Model file for the job. Use its own axes, mm. Face numbers are marked on the shaded views. Coordinates: 2 decimals unless noted, no trailing zeros. Write each loop counter-clockwise with the first axis right and the second up, starting at its lowest first coordinate (ties: lowest second). Pieces come first, ordered by that corner, then holes. Notation, with made-up numbers: (-18, 29) -> (11, 29) arc R15 cw to (11, 45) -> close; hole circle Ø11 at (2, 11). An arc over 180 degrees is marked (long way). Answer as a JSON object with one key per item and string values. Group by question number.
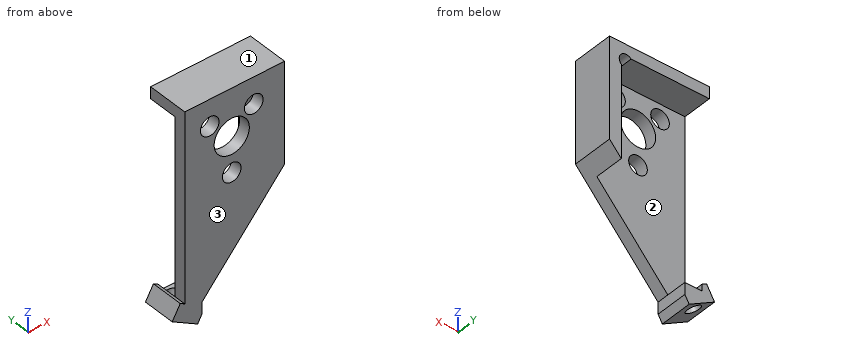
from build123d import *

# Parameters (mm, degrees)
SKETCH1_W                     = 8.5
SKETCH1_H                     = 17.5
BOSS_EXTRUDE1_DEPTH           = 3.5
SKETCH2_W                     = 6.5
SKETCH2_H                     = 15.5
CUT_EXTRUDE1_DEPTH            = 2.5
SKETCH3_R                     = 1.5
GRIN_HOLE_DEPTH               = 2
SKETCH6_R                     = 0.5953125
CORNER_DIVOT_DEPTH            = 2.5
SKETCH7_R                     = 0.79375
MAGNET_HOLES_DEPTH            = 2
BOSS_EXTRUDE2_DEPTH           = 3.5
SKETCH14_W                    = 5.965258944
SKETCH14_H                    = 5.132960456
SET_SCREW_EXTENSION_DEPTH     = 0.75
TAP_DRILL_FOR_0_80_TAP1_D     = 1.19126
TAP_DRILL_FOR_0_80_TAP1_DEPTH = 7.11
TAP_DRILL_FOR_0_80_TAP1_TIP   = 0.357890611
DIAGONAL_CUT_DEPTH            = 5
SKETCH16_W                    = 1
SKETCH16_H                    = 15.5
VERTICAL_CUT_DEPTH            = 3


with BuildPart() as part:
    # Sketch1 → Boss-Extrude1 (new body)
    with BuildSketch(Plane(origin=(0, 0, 0), x_dir=(1, 0, 0), z_dir=(0, 1, 0))):
        Rectangle(SKETCH1_W, SKETCH1_H)
    extrude(amount=BOSS_EXTRUDE1_DEPTH)

    # Sketch2 → Cut-Extrude1 (cut)
    with BuildSketch(Plane(origin=(0, 3.5, 0), x_dir=(1, 0, 0), z_dir=(0, 1, 0))):
        Rectangle(SKETCH2_W, SKETCH2_H)
    extrude(amount=-CUT_EXTRUDE1_DEPTH, mode=Mode.SUBTRACT)

    # Sketch3 → GRIN Hole (cut, through all)
    with BuildSketch(Plane(origin=(0, 1, 0), x_dir=(1, 0, 0), z_dir=(0, 1, 0))):
        with Locations((-0.25, -4.75)):
            Circle(SKETCH3_R)
    extrude(amount=-GRIN_HOLE_DEPTH, mode=Mode.SUBTRACT)

    # Sketch6 → Corner divot (cut)
    with BuildSketch(Plane(origin=(0, 3.5, 0), x_dir=(1, 0, 0), z_dir=(0, 1, 0))):
        with Locations((2.829050494, -7.329050494)):
            Circle(SKETCH6_R)
    extrude(amount=-CORNER_DIVOT_DEPTH, mode=Mode.SUBTRACT)

    # Sketch7 → Magnet Holes (cut, through all)
    with BuildSketch(Plane(origin=(0, 1, 0), x_dir=(1, 0, 0), z_dir=(0, 1, 0))):
        with Locations((-0.25, -1.75)):
            Circle(SKETCH7_R)
        with Locations((-2.125, -6.5)):
            Circle(SKETCH7_R)
        with Locations((1.625, -6.5)):
            Circle(SKETCH7_R)
    extrude(amount=-MAGNET_HOLES_DEPTH, mode=Mode.SUBTRACT)

    # Sketch9 → Boss-Extrude2 (add)
    with BuildSketch(Plane(origin=(0, 3.5, 0), x_dir=(1, 0, 0), z_dir=(0, 1, 0))):
        Polygon((-3.153871189, 9.382850264), (-5.318934698, 8.132850264), (-4.635921996, 6.949837562), (-4.021927306, 7.304327562), (-3.084853178, 7.845347562), (-2.470858487, 8.199837562), align=None)
    extrude(amount=-BOSS_EXTRUDE2_DEPTH)

    # Sketch14 → Set Screw Extension (cut)
    with BuildSketch(Plane(origin=(0, 3.5, 0), x_dir=(1, 0, 0), z_dir=(0, 1, 0))):
        with Locations((-3.25, 7.75)):
            Rectangle(SKETCH14_W, SKETCH14_H)
    extrude(amount=-SET_SCREW_EXTENSION_DEPTH, mode=Mode.SUBTRACT)

    # Tap Drill for #0-80 Tap1
    with Locations(Plane(origin=(-4.851361142, 0, -8.402803983), x_dir=(-0.866025404, 0, 0.5), z_dir=(-0.5, 0, -0.866025404))):
        with Locations((-0.710092562, 1.875)):
            Hole(TAP_DRILL_FOR_0_80_TAP1_D / 2, depth=TAP_DRILL_FOR_0_80_TAP1_DEPTH)
            with Locations((0, 0, -(TAP_DRILL_FOR_0_80_TAP1_DEPTH + TAP_DRILL_FOR_0_80_TAP1_TIP / 2))):  # 118° drill point
                Cone(0, TAP_DRILL_FOR_0_80_TAP1_D / 2, TAP_DRILL_FOR_0_80_TAP1_TIP, mode=Mode.SUBTRACT)

    # Sketch15 → Diagonal Cut (cut)
    with BuildSketch(Plane(origin=(0, 0, 0), x_dir=(1, 0, 0), z_dir=(0, 1, 0))):
        Polygon((-2.788494918, 9.313235547), (-2.788494918, 7.75), (4.25, -0.208562074), (4.25, 9.313235547), align=None)
    extrude(amount=DIAGONAL_CUT_DEPTH, mode=Mode.SUBTRACT)

    # Sketch16 → Vertical Cut (cut)
    with BuildSketch(Plane(origin=(0, 1, 0), x_dir=(1, 0, 0), z_dir=(0, 1, 0))):
        with Locations((-3.75, 0)):
            Rectangle(SKETCH16_W, SKETCH16_H)
    extrude(amount=VERTICAL_CUT_DEPTH, mode=Mode.SUBTRACT)


solid = part.part
(1) Cut at A-A on z = 6.5. List the corners of the cut face in (x, y), plus the area to 4 significant figures.
(2) Pull direction Z, two halves, no side cores. Call the marked faces 1, 2 and 3: released by +Z, released by -Z, zero draft, split by the parting line, or undercut.
(3) Cut at C-C on y = 3.1. List the corners of the cut face in (x, z).
(4) Cut at D-D on x = 2. List the corners of the cut face in (y, z), plus the area to 3 significant figures.
(5) Cut at B-B on z = 1.75. List the corners of the cut face in (x, y), plus the area to 3 significant figures.
(6) Pin check, flat tips, straight feed: pin 1 (1.2 mm diameter, centred on y = 2, z = 4, fed in from -X); pin 2 (0.7 mm diameter, centred on x = -3.5, z = -8, fed in from +Y); pin 3 (0.5 mm diameter, centred on y = 2, z = -8.5, fed in from +X). Stop position of each tip, or through.
(7) Wall check: probe 1 along X at (y, z) = (0.6, 6.5); probe 2 along Z at (x, y) = (-0.25, 0.35); probe 3 along X at (y, z) = (0.75, 1.75). Give the ranges that are in metal, low to high.
Results found:
{
 "1": {"outline": "(-4.25, 0) -> (-2.92, 0) -> (-2.92, 1) -> (-4.25, 1) -> close; (-1.33, 0) -> (0.83, 0) -> (0.83, 1) -> (-1.33, 1) -> close; (2.42, 0) -> (4.25, 0) -> (4.25, 3.5) -> (3.25, 3.5) -> (3.25, 1) -> (2.42, 1) -> close", "area": "7.825 mm²"},
 "2": {"face 1": "released by +Z", "face 2": "undercut", "face 3": "zero draft"},
 "3": {"outline": "(-4.25, 7.75) -> (2.41, 7.75) arc R0.6 cw to (3.25, 6.91) -> (3.25, -0.92) -> (4.25, 0.21) -> (4.25, 8.75) -> (-4.25, 8.75) -> close"},
 "4": {"outline": "(0, -2.34) -> (1, -2.34) -> (1, 5.8) -> (0, 5.8) -> close; (0, 7.2) -> (1, 7.2) -> (1, 7.75) -> (3.5, 7.75) -> (3.5, 8.75) -> (0, 8.75) -> close", "area": "12.2 mm²"},
 "5": {"outline": "(-4.25, 0) -> (-1.04, 0) -> (-1.04, 1) -> (-4.25, 1) -> close; (0.54, 0) -> (4.25, 0) -> (4.25, 3.5) -> (3.25, 3.5) -> (3.25, 1) -> (0.54, 1) -> close", "area": "9.41 mm²"},
 "6": {"pin 1": "stops at x = 3.25", "pin 2": "stops at y = 2.75", "pin 3": "stops at x = -2.79"},
 "7": {"probe 1": "x = -4.25 to -2.92, -1.33 to 0.83, 2.42 to 4.25", "probe 2": "z = -4.88 to 0.96, 2.54 to 3.25, 6.25 to 8.75", "probe 3": "x = -4.25 to -1.04, 0.54 to 4.25"}
}
